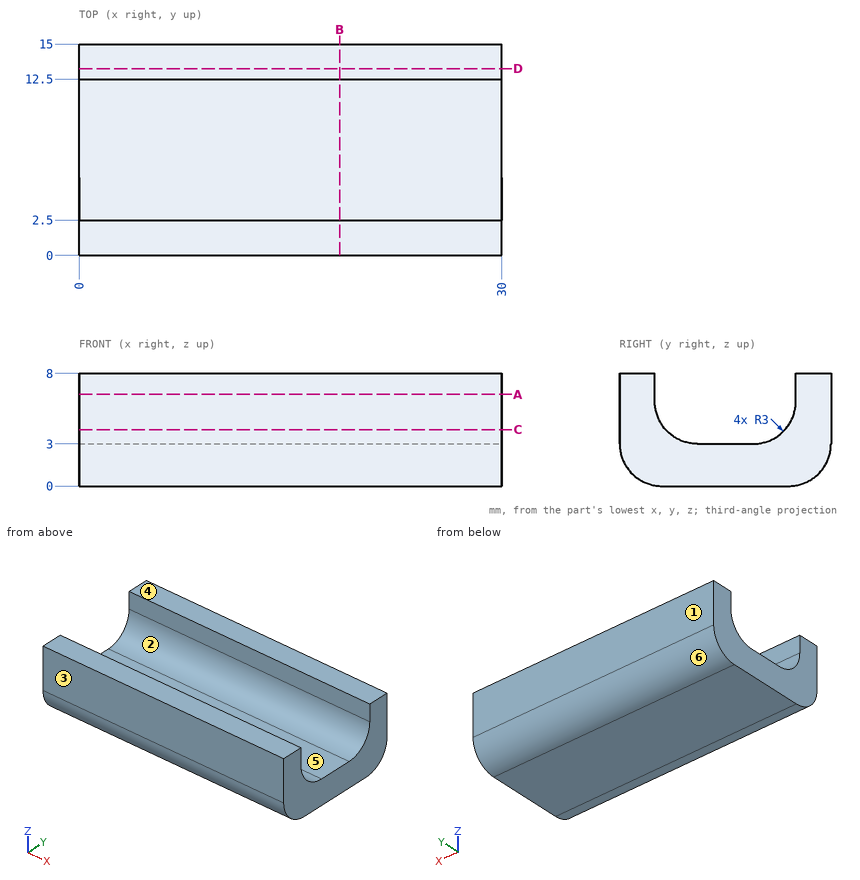
Source: three-view drawing plus pictorial views. Frame: mm from the lowest corner of the part. A direction names the side the tool comes from. Round coordinates to 2 decimals unless told otherwise and drop trailing zeros. Write each loop counter-clockwise with the first axis right and the second up, starting at its lowest first coordinate (ties: lowest second). Pieces come first, ordered by that corner, then holes. Notation, with made-up numbers: (-4.5, 64) -> (45.5, 64) arc R14 ccw to (45.5, 91) -> close; hole circle Ø3 at (46.25, 81). An arc over 180 degrees is marked (long way). Return JSON: item names as keys, results as strings.
Q1. Mould query, pull axis Y, two halves, no side actions, for the marked faces 3, 4, 5 and 6. Classes: +Y half, -Y half, draft (parallel to the pull), parting line (faces both ways), or undercut.
From the geometry:
{"face 3": "-Y half", "face 4": "draft", "face 5": "undercut", "face 6": "+Y half"}
Q2. First-contact query: pin 1 Ø3 at (x, y) = (21, 7.5) entering from +Z. Flat tip, straight axial feed; report the tip coordinate or a pass-through.
From the geometry:
{"pin 1": "z = 3"}
Q3. Section D-D on y = 13.25. Return the cut outline in (x, z), and give its area (3 significant figures).
From the geometry:
{"outline": "(0, 0.27) -> (30, 0.27) -> (30, 8) -> (0, 8) -> close", "area": "232 mm2"}
Q4. Section B-B on x = 18.5. Return the cut outline in (y, z), and give its area (3 significant figures).
From the geometry:
{"outline": "(0, 3) arc R3 ccw to (3, 0) -> (12, 0) arc R3 ccw to (15, 3) -> (15, 8) -> (12.5, 8) -> (12.5, 6) arc R3 cw to (9.5, 3) -> (5.5, 3) arc R3 cw to (2.5, 6) -> (2.5, 8) -> (0, 8) -> close", "area": "70.0 mm2"}
Q5. Ray query, line 1 (Y direction, x = 11.75, z = 7.5); line 2 (Y direction, x = 26.75, z = 3.25); line 3 (Z direction, x = 7, y = 7.5). Return the intervals inside material, ascending.
From the geometry:
{"line 1": "0 to 2.5, 12.5 to 15", "line 2": "0 to 4.3, 10.7 to 15", "line 3": "0 to 3"}
Q6. Set-up query: the marked faces 1 and 2. Return all of +Z, -Z, +X, -X, +Y, -Y with unobstructed straight access to the full face (end or side cutting, diameter ignored); none if empty.
From the geometry:
{"face 1": "+Z, -Z, +X, -X, +Y", "face 2": "+Z, +X, -X"}
Q7. Section C-C on z = 4. Return the cut outline in (x, y).
From the geometry:
{"outline": "(0, 0) -> (30, 0) -> (30, 3.26) -> (0, 3.26) -> close; (0, 11.74) -> (30, 11.74) -> (30, 15) -> (0, 15) -> close"}
Q8. Section A-A on z = 6.5. Return the cut outline in (x, y).
From the geometry:
{"outline": "(0, 0) -> (30, 0) -> (30, 2.5) -> (0, 2.5) -> close; (0, 12.5) -> (30, 12.5) -> (30, 15) -> (0, 15) -> close"}
